```python
from build123d import *

# Parameters (mm, degrees)
SKETCH2_W            = 800
SKETCH2_H            = 300
BOSS_EXTRUDE1_DEPTH  = 100
SKETCH3_W            = 50
SKETCH3_H            = 50
BOSS_EXTRUDE2_DEPTH  = 200
SKETCH4_W            = 800
SKETCH4_H            = 300
SKETCH4_W_2          = 700
SKETCH4_H_2          = 200
BOSS_EXTRUDE3_DEPTH  = 150
SKETCH5_W            = 85.954447183
SKETCH5_H            = 200
CUT_EXTRUDE1_DEPTH   = 750
SKETCH6_W            = 7
SKETCH6_H            = 200
BOSS_EXTRUDE5_DEPTH  = 185
SKETCH9_W            = 7
SKETCH9_H            = 192.990182273
BOSS_EXTRUDE6_DEPTH  = 160
SKETCH12_W           = 200
SKETCH12_H           = 200
CUT_EXTRUDE4_DEPTH   = 111
SKETCH14_W           = 6.809905138
SKETCH14_H           = 7.009817727
BOSS_EXTRUDE9_DEPTH  = 160
BOSS_EXTRUDE10_DEPTH = 7
F_3DSKETCH2_R        = 2.5
CUT_EXTRUDE5_DEPTH   = 263.5


with BuildPart() as part:
    # Sketch2 → Boss-Extrude1 (new body)
    with BuildSketch(Plane.XY):
        with Locations((52.951699463, -18.694096601)):
            Rectangle(SKETCH2_W, SKETCH2_H)
    extrude(amount=BOSS_EXTRUDE1_DEPTH)

    # Sketch3 → Boss-Extrude2 (add)
    with BuildSketch(Plane.XY.offset(100)):
        with Locations((-322.048300537, 106.305903399)):
            Rectangle(SKETCH3_W, SKETCH3_H)
        with Locations((-322.048300537, -143.694096601)):
            Rectangle(SKETCH3_W, SKETCH3_H)
        with Locations((427.951699463, 106.305903399)):
            Rectangle(SKETCH3_W, SKETCH3_H)
        with Locations((427.951699463, -143.694096601)):
            Rectangle(SKETCH3_W, SKETCH3_H)
    extrude(amount=BOSS_EXTRUDE2_DEPTH)

    # Sketch4 → Boss-Extrude3 (add)
    with BuildSketch(Plane(origin=(0, 0, 0), x_dir=(-1, 0, 0), z_dir=(0, 0, -1))):
        with Locations((-52.951699463, -18.694096601)):
            Rectangle(SKETCH4_W, SKETCH4_H)
        with Locations((-52.951699463, -18.694096601)):
            Rectangle(SKETCH4_W_2, SKETCH4_H_2, mode=Mode.SUBTRACT)
    extrude(amount=BOSS_EXTRUDE3_DEPTH)

    # Sketch5 → Cut-Extrude1 (cut)
    with BuildSketch(Plane(origin=(452.951699463, 0, 0), x_dir=(0, 0, -1), z_dir=(1, 0, 0))):
        with Locations((-27.022776409, -18.694096601)):
            Rectangle(SKETCH5_W, SKETCH5_H)
    extrude(amount=-CUT_EXTRUDE1_DEPTH, mode=Mode.SUBTRACT)

    # Sketch6 → Boss-Extrude5 (add)
    with BuildSketch(Plane(origin=(0, 0, 70), x_dir=(-1, 0, 0), z_dir=(0, 0, -1))):
        with Locations((73.548300537, -18.694096601)):
            Rectangle(SKETCH6_W, SKETCH6_H)
    extrude(amount=BOSS_EXTRUDE5_DEPTH)

    # Sketch9 → Boss-Extrude6 (add)
    with BuildSketch(Plane(origin=(0, 0, 70), x_dir=(-1, 0, 0), z_dir=(0, 0, -1))):
        with Locations((-153.451699463, -15.189187737)):
            Rectangle(SKETCH9_W, SKETCH9_H)
    extrude(amount=BOSS_EXTRUDE6_DEPTH)

    # Sketch12 → Cut-Extrude4 (cut)
    with BuildSketch(Plane(origin=(0, 0, 70), x_dir=(-1, 0, 0), z_dir=(0, 0, -1))):
        with Locations((197.048300537, -18.694096601)):
            Rectangle(SKETCH12_W, SKETCH12_H)
        with Locations((-29.951699463, -18.694096601)):
            Rectangle(SKETCH12_W, SKETCH12_H)
    extrude(amount=-CUT_EXTRUDE4_DEPTH, mode=Mode.SUBTRACT)

    # Sketch14 → Boss-Extrude9 (add)
    with BuildSketch(Plane(origin=(0, 0, 70), x_dir=(-1, 0, 0), z_dir=(0, 0, -1))):
        with Locations((-153.546746894, -115.189187738)):
            Rectangle(SKETCH14_W, SKETCH14_H)
    extrude(amount=BOSS_EXTRUDE9_DEPTH)

    # 3DSketch1 → Boss-Extrude10 (add)
    with BuildSketch(Plane(origin=(-297.048300537, 81.305903399, -150), x_dir=(-0.033314830232638246, -0.9994449069791543, 0), z_dir=(0, 0, -1))):
        Polygon((0, 0), (0.233203812, 6.996114349), (-9.761245258, 7.329262651), (-9.99444907, 0.333148302), align=None)
        Polygon((199.888981396, -6.662966047), (200.122185207, 0.333148302), (210.116634277, 0), (209.883430466, -6.996114349), align=None)
    extrude(amount=BOSS_EXTRUDE10_DEPTH)

    # 3DSketch2 → Cut-Extrude5 (cut, symmetric)
    with BuildSketch(Plane(origin=(-297.048300537, -128.694096601, -157), x_dir=(-0.7071067811865476, 0, 0.7071067811865476), z_dir=(0, -1, 0))):
        with Locations(Location((4.949747468, 0, 0), (0, 0, 135))):
            Circle(F_3DSKETCH2_R)
    extrude(amount=CUT_EXTRUDE5_DEPTH, both=True, mode=Mode.SUBTRACT)


solid = part.part
```
For this review, take the finished solid that the model builds, in its own axes (mm). A direction names the side the tool comes from. Coordinates: 2 decimals unless noted, no trailing zeros. Write each loop counter-clockwise with the first axis right and the second up, starting at its lowest first coordinate (ties: lowest second). Pieces come first, ordered by that corner, then holes. Notation, with made-up numbers: (46, 17.25) -> (88, 17.25) arc R18 cw to (88, 27.25) -> close; hole circle Ø7 at (-12.75, -37). An arc over 180 degrees is marked (long way). Put each result on its own line as item: value.
Q1. Take a section at C-C, the plane z = 169.5. State the section outline as (x, y) points, then the cut area to 3 significant figures.
From the geometry:
outline: (-347.05, -168.69) -> (-297.05, -168.69) -> (-297.05, -118.69) -> (-347.05, -118.69) -> close; (-347.05, 81.31) -> (-297.05, 81.31) -> (-297.05, 131.31) -> (-347.05, 131.31) -> close; (402.95, -168.69) -> (452.95, -168.69) -> (452.95, -118.69) -> (402.95, -118.69) -> close; (402.95, 81.31) -> (452.95, 81.31) -> (452.95, 131.31) -> (402.95, 131.31) -> close
area: 10,000 mm2
Q2. Tool access review of faces 4 (the flat face through (-297.048, -144, 199)), 5 (the flat face through (-297.048, -20, -23)), 6 (the flat face through (156.952, -20, -9)): name each direction out of +Z, -Z, +X, -X, +Y, -Y from which nothing blocks a thin tool from reaching the whole face with its end or side.
From the geometry:
face 4: +Z, +Y, -Y
face 5: +Z, -Z
face 6: -Z
Q3. Take a section at B-B, the plane y = -64. State the section outline as (x, z) points, then the cut area to 3 significant figures.
From the geometry:
outline: (-347.05, -150) -> (-297.05, -150) -> (-297.05, 100) -> (-347.05, 100) -> close; (-97.05, 70) -> (-77.05, 70) -> (-77.05, -115) -> (-70.05, -115) -> (-70.05, 100) -> (-97.05, 100) -> close; (129.95, 70) -> (149.95, 70) -> (149.95, -90) -> (156.95, -90) -> (156.95, 70) -> (452.95, 70) -> (452.95, 100) -> (129.95, 100) -> close; (402.95, -150) -> (452.95, -150) -> (452.95, -15.95) -> (402.95, -15.95) -> close
area: 32,100 mm2
Q4. Clearance check with flat-ended pins moving along their axes: pin 1 Ø7.5 at (x, y) = (-74, -30) entering from -Z; pin 2 Ø6 at (x, y) = (137.5, -42) entering from -Z; pin 3 Ø15 at (x, y) = (-317, -11) entering from +Z. State where each tip first meets the part, or that it passes through.
From the geometry:
pin 1: stops at z = -115
pin 2: stops at z = 70
pin 3: stops at z = 100
Q5. The part is to be moulded in two halves that separate along X. For faces 1 (the flat face through (428, 81.306, 199)), 2 (the flat face through (452.952, -21, -22)), 3 (the flat face through (-77.048, -20, -21)), say which applies: +X half, -X half, draft (parallel to the pull), parting line (faces both ways), or undercut.
From the geometry:
face 1: draft
face 2: +X half
face 3: undercut
Q6. Wall thickness on L1, parallel to X at y = 39.5, z = 93.5; L2, parallel to X at y = -21.5, z = 40; L3, parallel to Y at x = -208, z = -102: over which ranges is each line inside the solid? List them lowest first.
From the geometry:
L1: x = -347.05 to -297.05, -97.05 to -70.05, 129.95 to 452.95
L2: x = -347.05 to -297.05, -77.05 to -70.05, 149.95 to 156.95
L3: y = -168.69 to -118.69, 81.31 to 131.31
Q7. Take a section at A-A, the plane x = 5. State the section outline as (y, z) points.
From the geometry:
outline: (-168.69, -150) -> (-118.69, -150) -> (-118.69, 100) -> (-168.69, 100) -> close; (81.31, -150) -> (131.31, -150) -> (131.31, 100) -> (81.31, 100) -> close
Q8. Take a section at D-D, the plane z = -47. State the section outline as (x, y) points.
From the geometry:
outline: (-347.05, -168.69) -> (452.95, -168.69) -> (452.95, 131.31) -> (-347.05, 131.31) -> close; hole (-297.05, -118.69) -> (-77.05, -118.69) -> (-77.05, 81.31) -> (-297.05, 81.31) -> close; hole (-70.05, -118.69) -> (150.14, -118.69) -> (150.14, -111.68) -> (149.95, -111.68) -> (149.95, 81.31) -> (-70.05, 81.31) -> close; hole (156.95, -118.69) -> (402.95, -118.69) -> (402.95, 81.31) -> (156.95, 81.31) -> close
